Could you check a few things on this drawing? It's one solid part, dimensions in mm from its lowest x, y, z. A direction names the side the tool comes from. Give positions to 0.01 mm unless a question says otherwise; leave off trailing zeros. Loops run counter-clockwise (first coordinate to the right, second up) from the corner with the lowest first, then second, coordinate; pieces in that order, holes last. Notation, with made-up numbers: (76.25, 35.5) -> (104.25, 35.5) arc R9 ccw to (104.25, 40.5) -> close; hole circle Ø2 at (14.5, 35.5). An arc over 180 degrees is marked (long way). One line per question, with ' | ' between items.
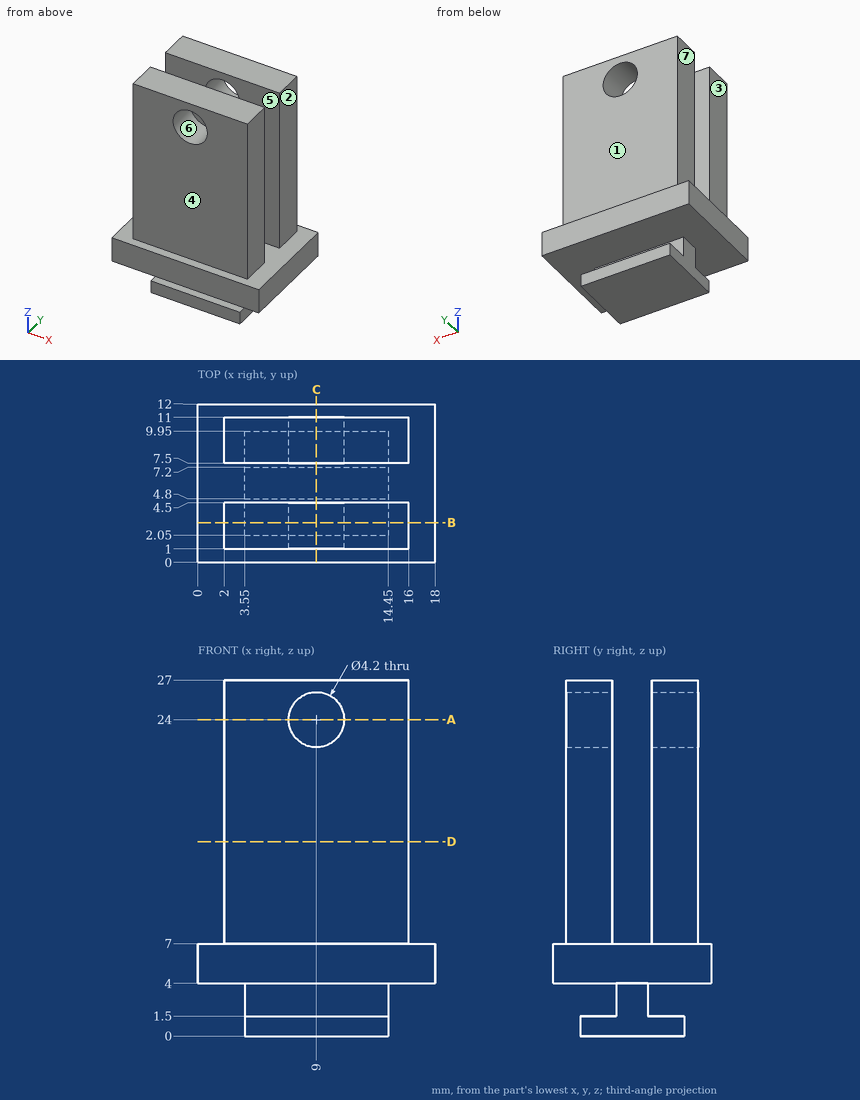
Q1. If we section it at D-D (z = 14.75): Write out the boundary of the cut face in (x, y), plus the area to 3 significant figures.
Entries:
outline: (2, 1) -> (16, 1) -> (16, 4.5) -> (2, 4.5) -> close; (2, 7.5) -> (16, 7.5) -> (16, 11) -> (2, 11) -> close | area: 98.0 mm²
Q2. If we section it at B-B (y = 3): Write out the boundary of the cut face in (x, z).
Entries:
outline: (0, 4) -> (18, 4) -> (18, 7) -> (16, 7) -> (16, 27) -> (2, 27) -> (2, 7) -> (0, 7) -> close; (3.55, 0) -> (14.45, 0) -> (14.45, 1.5) -> (3.55, 1.5) -> close; hole circle Ø4.2 at (9, 24)
Q3. On a 3-axis mill with a long thin cutter (end or side, diameter ignored), from which of +Z, -Z, +X, -X, +Y, -Y can I reach the whole of each face in a straight line? I mean the marked faces 1, 2, 3 and 4. Say none if no direction works.
Entries:
face 1: +Z, +X, -X, +Y | face 2: +Z, +X, +Y, -Y | face 3: +Z, -X, +Y, -Y | face 4: +Z, +X, -X, -Y
Q4. If we section it at C-C (x = 9): Write out the boundary of the cut face in (y, z).
Entries:
outline: (0, 4) -> (4.8, 4) -> (4.8, 1.5) -> (2.05, 1.5) -> (2.05, 0) -> (9.95, 0) -> (9.95, 1.5) -> (7.2, 1.5) -> (7.2, 4) -> (12, 4) -> (12, 7) -> (11, 7) -> (11, 21.9) -> (7.5, 21.9) -> (7.5, 7) -> (4.5, 7) -> (4.5, 21.9) -> (1, 21.9) -> (1, 7) -> (0, 7) -> close; (1, 26.1) -> (4.5, 26.1) -> (4.5, 27) -> (1, 27) -> close; (7.5, 26.1) -> (11, 26.1) -> (11, 27) -> (7.5, 27) -> close
Q5. If we mould it in two halves opening along X, with no side actions, what happens to the marked faces 5, 6 and 7? For each: pulls with the +X half, pulls with the -X half, needs draft (parallel to the pull), parting line crosses it, or undercut.
Entries:
face 5: needs draft | face 6: undercut | face 7: pulls with the -X half
Q6. For pin 1 Ø4 at (x, z) = (9.5, 18.5) entering from -Y; pin 2 Ø2 at (x, z) = (7.5, 3.5) entering from -Y; pin 3 Ø3.5 at (x, z) = (9, 24) entering from -Y; pin 4 Ø3 at (y, z) = (3, 9) entering from +X, each with a flat end and sliding along its axis, tell me the tip position at first contact or that it passes through.
Entries:
pin 1: y = 1 | pin 2: y = 0 | pin 3: through | pin 4: x = 16
Q7. If we section it at A-A (z = 24): Write out the boundary of the cut face in (x, y), plus the area to 3 significant figures.
Entries:
outline: (2, 1) -> (6.9, 1) -> (6.9, 4.5) -> (2, 4.5) -> close; (2, 7.5) -> (6.9, 7.5) -> (6.9, 11) -> (2, 11) -> close; (11.1, 1) -> (16, 1) -> (16, 4.5) -> (11.1, 4.5) -> close; (11.1, 7.5) -> (16, 7.5) -> (16, 11) -> (11.1, 11) -> close | area: 68.6 mm²
Q8. If I drill on probe 1 along Z at (x, y) = (9, 8.6); probe 2 along Z at (x, y) = (12.25, 4); probe 3 along Y at (x, z) = (13, 17.5), over which ranges is the centre line in solid material (lowest first)? Write a range as from..to.
Entries:
probe 1: 0..1.5, 4..21.9, 26.1..27 | probe 2: 0..1.5, 4..27 | probe 3: 1..4.5, 7.5..11
